The model under review builds one solid part; all positions refer to its coordinate system, in mm. A direction names the side the tool comes from. Round coordinates to 2 decimals unless told otherwise and drop trailing zeros. Order: outer loops, then holes, each group sorted by start corner. A loop starts at its lowest first (then second) coordinate and runs counter-clockwise, first axis right, second up. Notation, with made-up numbers: M -29,42 L 2,42 A26 cw 2,67 Z; hole C 42.5,19 d5. An arc over 180 degrees is marked long. Use a Markdown table: item, result. Add a question column.
1. To check wall thickness, follow probe 1 along Y at (x, z) = (1785, 42.5); probe 2 along X at (y, z) = (-16, 42.5); probe 3 along X at (y, z) = (-18, 52). State the ranges of each line that lie inside material, in increasing order.
2. For faces 1 (the flat face through (697, -241.3, 52)), 2 (the flat face through (1349, -36, 101.6)), 3 (the flat face through (2572, -38.1, 63)), list the 3-axis set-ups (+Z, -Z, +X, -X, +Y, -Y) from which the entire face can be reached by the end or side of a thin tool; tool diameter is ignored.
3. Consider section B-B on y = -153.5. State the section outline as (x, z) points, then the cut area to 3 significant figures.
4. Insertion check: P1, Ø21.5, axis at x = 2574.5, z = 46, coming from the +Y side; P2, Ø10, axis at y = -39.5, z = 20, coming from the +X side; P3, Ø2, axis at y = -247.5, z = 34, coming from the -X side. Each pin has a flat end and moves straight along its axis. Give the tip position at first contact, or say it passes through.
5. Consider section A-A on x = 2015. State the section outline as (y, z) points.
6. Consider section C-C on z = 24.5. Count the separate pieces of the cut face and the enclosed holes in it, then the cut area to 3 significant figures.
from build123d import *

# Parameters (mm, degrees)
F1_DEPTH = 38.1
F2_W     = 38.1
F2_H     = 101.6
F3_DEPTH = 203.2
F4_W     = 38.1
F4_H     = 101.6
F5_DEPTH = 38.1


# Not quite as in the source:
# - a feature names something its author has since deleted; it is built from what else it names


with BuildPart() as f1:
    # F0 (on Front) → F1 (new body)
    with BuildSketch(Plane.XZ):
        Polygon((71.1410858821, 101.6), (0, 0), (2544.7625, 0), (2615.9035858821, 101.6), align=None)
    extrude(amount=F1_DEPTH)

    # F2 (on face) → F3 (join)
    with BuildSketch(Plane.XZ.offset(38.1)):
        with Locations((90.1910858821, 50.8)):
            Rectangle(F2_W, F2_H)
        with Locations((496.5910858821, 50.8)):
            Rectangle(F2_W, F2_H)
        with Locations((902.9910858821, 50.8)):
            Rectangle(F2_W, F2_H)
        with Locations((1306.5125, 50.8)):
            Rectangle(F2_W, F2_H)
        with Locations((1712.9125, 50.8)):
            Rectangle(F2_W, F2_H)
        with Locations((2119.3125, 50.8)):
            Rectangle(F2_W, F2_H)
        with Locations((2525.7125, 50.8)):
            Rectangle(F2_W, F2_H)
    extrude(amount=F3_DEPTH)

    # F4 (on face) → F5 (join)
    with BuildSketch(Plane.XZ.offset(241.3)):
        Polygon((2615.9035858821, 101.6), (109.2410858821, 101.6), (109.2410858821, 0), (2544.7625, 0), align=None)
        with Locations((90.1910858821, 50.8)):
            Rectangle(F4_W, F4_H)
        Polygon((71.1410858821, 101.6), (0, 0), (71.1410858821, 0), align=None)
    extrude(amount=F5_DEPTH)


solid = f1.part
Answer block:
| question | item | result |
|---|---|---|
| 1 | probe 1 | -279.4 to -241.3, -38.1 to 0 |
| 1 | probe 2 | 29.76 to 2574.52 |
| 1 | probe 3 | 36.41 to 2581.17 |
| 2 | face 1 | +Z, -Z |
| 2 | face 2 | +Z, +X, -X, +Y, -Y |
| 2 | face 3 | +Z, -Z, +X |
| 3 | outline | M 71.14,0 L 109.24,0 L 109.24,101.6 L 71.14,101.6 Z; M 477.54,0 L 515.64,0 L 515.64,101.6 L 477.54,101.6 Z; M 883.94,0 L 922.04,0 L 922.04,101.6 L 883.94,101.6 Z; M 1287.46,0 L 1325.56,0 L 1325.56,101.6 L 1287.46,101.6 Z; M 1693.86,0 L 1731.96,0 L 1731.96,101.6 L 1693.86,101.6 Z; M 2100.26,0 L 2138.36,0 L 2138.36,101.6 L 2100.26,101.6 Z; M 2506.66,0 L 2544.76,0 L 2544.76,101.6 L 2506.66,101.6 Z |
| 3 | area | 27,100 mm^2 |
| 4 | P1 | y = 0 |
| 4 | P2 | x = 2562.13 |
| 4 | P3 | x = 23.11 |
| 5 | outline | M -279.4,0 L -241.3,0 L -241.3,101.6 L -279.4,101.6 Z; M -38.1,0 L 0,0 L 0,101.6 L -38.1,101.6 Z |
| 6 | separate pieces | 1 |
| 6 | enclosed holes | 6 |
| 6 | area | 248,000 mm^2 |
